Check sheet for the modelled part. Datum: model origin and axes. Units: mm. A direction names the side the tool comes from. Round coordinates to 2 decimals unless told otherwise and drop trailing zeros. Write each loop counter-clockwise with the first axis right and the second up, starting at its lowest first coordinate (ties: lowest second). Pieces come first, ordered by that corner, then holes. Notation, with made-up numbers: (-35, -21.75) - (-10, -21.75) arc R23 cw to (-10, -0.75) - close; hole circle Ø11 at (64, -23). An arc over 180 degrees is marked (long way). Answer as a JSON object with one key per item and string values. Group by question number.
Item 1: Sectioned sample at D-D on y = 2. Record the boundary of the cut face in (x, z) (3 decimals).
Item 2: Set-up check for faces 1 (the flat face through (0.5, 28.62, -2.33)), 2 (the cylindrical face through (-3.78, 28.53, 2.9)): record each of +Z, -Z, +X, -X, +Y, -Y from which the full face is reachable in a straight line by a thin tool's end or side.
Item 3: Sectioned sample at A-A on y = 27.5. Record the boundary of the cut face in (x, z) (1 decimal), plus the area to 3 significant figures.
Item 4: Gauge pin test, flat ends, axial feed: P1, Ø4, axis at x = -1.5, y = 10, coming from the +Z side (3 decimals); P2, Ø3, axis at x = 0, z = 2, coming from the -Y side; P3, Ø1.5, axis at y = 22.5, z = 1, coming from the +X side. Record the tip position at first contact, or that the pin passes through.
Item 5: Sectioned sample at B-B on x = 1.5. Record the boundary of the cut face in (y, z).
Item 6: Thickness scan on line 1 (Y direction, x = 4, z = -0.25); line 2 (Y direction, x = -1.75, z = -1.5); line 3 (Z direction, x = 0, y = 9.5) (3 decimals). Record the ranges inside material, lowest first.
Item 7: Release check for a two-part mould opening along Z. For faces 3 (the cylindrical face through (-0.69, 12.52, 3.1)), 4 (the flat face through (1.764, 28.619, 1.6)), 5 (the flat face through (0, 0, 0)) record: pulls with the +Z half, pulls with the -Z half, needs draft (parallel to the pull), parting line crosses it, or undercut.
```python
from build123d import *

# Parameters (mm, degrees)
SKETCH1_R           = 3.175
BOSS_EXTRUDE1_DEPTH = 25.4
SKETCH2_R           = 4.7625
BOSS_EXTRUDE2_DEPTH = 6.35
CUT_EXTRUDE1_DEPTH  = 6.35


with BuildPart() as part:
    # Sketch1 → Boss-Extrude1 (new body)
    with BuildSketch(Plane(origin=(0, 0, 0), x_dir=(1, 0, 0), z_dir=(0, 1, 0))):
        Circle(SKETCH1_R)
    extrude(amount=BOSS_EXTRUDE1_DEPTH)

    # Sketch2 → Boss-Extrude2 (add)
    with BuildSketch(Plane(origin=(0, 25.4, 0), x_dir=(1, 0, 0), z_dir=(0, 1, 0))):
        Circle(SKETCH2_R)
    extrude(amount=BOSS_EXTRUDE2_DEPTH)

    # Sketch3 → Cut-Extrude1 (cut)
    with BuildSketch(Plane(origin=(0, 31.75, 0), x_dir=(1, 0, 0), z_dir=(0, 1, 0))):
        Polygon((-2.692012499, 0.559944154), (-1.830932112, -2.051379134), (0.861080387, -2.611323288), (2.692012499, -0.559944154), (1.830932112, 2.051379134), (-0.861080387, 2.611323288), align=None)
    extrude(amount=-CUT_EXTRUDE1_DEPTH, mode=Mode.SUBTRACT)


solid = part.part
```
Completed:
{
 "1": {"outline": "circle Ø6.35 at (0, 0)"},
 "2": {"face 1": "+Y", "face 2": "+Y, -Y"},
 "3": {"outline": "circle Ø9.5 at (0, 0); hole (-2.7, -0.6) - (-0.9, -2.6) - (1.8, -2.1) - (2.7, 0.6) - (0.9, 2.6) - (-1.8, 2.1) - close", "area": "51.6 mm²"},
 "4": {"P1": "z = 3.175", "P2": "y = 0", "P3": "x = 3.17"},
 "5": {"outline": "(0, -2.8) - (25.4, -2.8) - (25.4, -4.52) - (31.75, -4.52) - (31.75, -2.12) - (25.4, -2.12) - (25.4, 1.9) - (31.75, 1.9) - (31.75, 4.52) - (25.4, 4.52) - (25.4, 2.8) - (0, 2.8) - close"},
 "6": {"line 1": "25.4 to 31.75", "line 2": "0 to 25.4", "line 3": "-3.175 to 3.175"},
 "7": {"face 3": "parting line crosses it", "face 4": "undercut", "face 5": "needs draft"}
}
